Verification items for the finished model (mm, model axes). Face numbers are marked on the shaded views. A direction names the side the tool comes from. Round coordinates to 2 decimals unless told otherwise and drop trailing zeros. Order: outer loops, then holes, each group sorted by start corner. A loop starts at its lowest first (then second) coordinate and runs counter-clockwise, first axis right, second up. Notation, with made-up numbers: (80, -39) -> (94, -39) arc R16 ccw to (94, -31) -> close; hole circle Ø5 at (-37, -11.75). An arc over 180 degrees is marked (long way). Return JSON: item names as keys, results as strings. Group by question number.
Item 1: Sectioned sample at C-C on x = 19.5. Record the cut outline in (y, z), plus the area to 3 significant figures.
Item 2: Depth check by flat-ended pin: pin 1 Ø1.4 at (x, y) = (17.46, 17.65) entering from -Z (3 decimals); pin 2 Ø2 at (x, z) = (8, 2.5) entering from -Y; pin 3 Ø3 at (x, y) = (6, 12.5) entering from -Z; pin 4 Ø1 at (x, z) = (19.5, 4) entering from -Y. Enter the tip coordinate at first touch or a pass-through.
Item 3: Sectioned sample at B-B on y = 11.75. Record the cut outline in (x, z).
Item 4: Scan lines: probe 1 along Y at (x, z) = (15.5, 1.85); probe 2 along Y at (x, z) = (18, 1.4); probe 3 along X at (y, z) = (11.75, 3.35). Record each from-to range of solid material in increasing order. Write a range as from..to.
Item 5: Access from +Z, -Z, +X, -X, +Y, -Y to the whole of each face (thin tool, end or side, straight path). Record for the marked faces 1, 2 and 3.
Item 6: Sectioned sample at D-D on y = 18.75. Record the cut outline in (x, z), plus the area to 3 significant figures.
Item 7: Sectioned sample at A-A on z = 1.45. Record the cut outline in (x, y).
Item 8: Draft check along Y on the marked faces 4, 5, 6 and 7. Enter one of: pulls with the +Y half, pulls with the -Y half, needs draft (parallel to the pull), parting line crosses it, or undercut.
```python
from build123d import *

# Parameters (mm, degrees)
BOSS_EXTRUDE1_DEPTH = 5
SKETCH3_R           = 2.75
JOINT_HOLE_DEPTH    = 32.253054869
CUT_EXTRUDE2_START  = 0.5
CUT_EXTRUDE2_DEPTH  = 5.5
SKETCH7_R           = 0.8
SCREW_HOLES_DEPTH   = 32.253054869
BOSS_EXTRUDE2_START = 5
SKETCH10_W          = 3.875984902
SKETCH10_H          = 3
BOSS_EXTRUDE2_DEPTH = 0.5


with BuildPart() as part:
    # Sketch1 → Boss-Extrude1 (new body)
    with BuildSketch(Plane.XY):
        with BuildLine():
            Line((22.456085085, 19.15366827), (11.355064571, 19.15366827))
            ThreePointArc((11.355064571, 19.15366827), (-0.543914915, 14.15366827), (11.355064571, 9.15366827))
            Line((11.355064571, 9.15366827), (22.456085085, 9.15366827))
            Line((22.456085085, 9.15366827), (22.456085085, 19.15366827))
        make_face()
    extrude(amount=BOSS_EXTRUDE1_DEPTH)

    # Sketch3 → Joint Hole (cut, through all)
    with BuildSketch(Plane.XY):
        with Locations((6.456085085, 14.15366827)):
            Circle(SKETCH3_R)
    extrude(amount=JOINT_HOLE_DEPTH, mode=Mode.SUBTRACT)

    # Sketch8 → Cut-Extrude2 (cut)
    with BuildSketch(Plane.XY.offset(CUT_EXTRUDE2_START)):
        with BuildLine():
            Line((15.231049473, 12.15366827), (22.456085085, 12.15366827))
            Line((22.456085085, 12.15366827), (22.456085085, 16.15366827))
            Line((22.456085085, 16.15366827), (15.231049473, 16.15366827))
            ThreePointArc((15.231049473, 16.15366827), (14.722457344, 17.712753782), (13.939399859, 19.15366827))
            Line((13.939399859, 19.15366827), (11.355064571, 19.15366827))
            ThreePointArc((11.355064571, 19.15366827), (13.456085085, 14.15366827), (11.355064571, 9.15366827))
            Line((11.355064571, 9.15366827), (13.939399859, 9.15366827))
            ThreePointArc((13.939399859, 9.15366827), (14.722457344, 10.594582758), (15.231049473, 12.15366827))
        make_face()
    extrude(amount=CUT_EXTRUDE2_DEPTH, mode=Mode.SUBTRACT)

    # Sketch7 → Screw Holes (cut, through all)
    with BuildSketch(Plane.XY):
        with Locations((17.456085085, 17.65366827)):
            Circle(SKETCH7_R)
        with Locations((17.456085085, 10.65366827)):
            Circle(SKETCH7_R)
    extrude(amount=SCREW_HOLES_DEPTH, mode=Mode.SUBTRACT)

    # Sketch10 → Boss-Extrude2 (add)
    with BuildSketch(Plane.XY.offset(BOSS_EXTRUDE2_START)):
        with Locations((13.293057022, 17.65366827)):
            Rectangle(SKETCH10_W, SKETCH10_H)
        with Locations((13.293057022, 10.65366827)):
            Rectangle(SKETCH10_W, SKETCH10_H)
    extrude(amount=-BOSS_EXTRUDE2_DEPTH)


solid = part.part
```
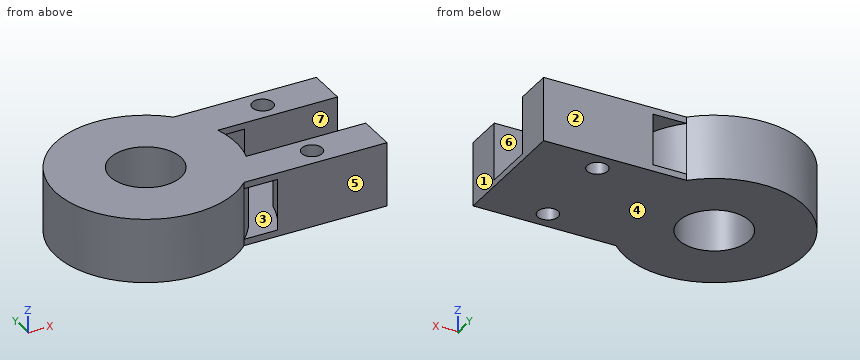
Recorded:
{
 "1": {"outline": "(9.15, 0) -> (19.15, 0) -> (19.15, 5) -> (16.15, 5) -> (16.15, 0.5) -> (12.15, 0.5) -> (12.15, 5) -> (9.15, 5) -> close", "area": "32.0 mm²"},
 "2": {"pin 1": "through", "pin 2": "y = 7.17", "pin 3": "z = 0", "pin 4": "y = 9.15"},
 "3": {"outline": "(-0.12, 0) -> (5.12, 0) -> (5.12, 5) -> (-0.12, 5) -> close; (7.79, 0) -> (22.46, 0) -> (22.46, 5) -> (7.79, 5) -> close; hole (13.03, 0.5) -> (15.13, 0.5) -> (15.13, 4.5) -> (13.03, 4.5) -> close"},
 "4": {"probe 1": "9.15..12.15, 16.15..19.15", "probe 2": "9.15..10.07, 11.24..12.15, 16.15..17.07, 18.24..19.15", "probe 3": "-0.12..5.12, 7.79..13.03, 15.13..22.46"},
 "5": {"face 1": "+Z, -Z, +X, +Y, -Y", "face 2": "+Z, -Z, +X, +Y", "face 3": "none"},
 "6": {"outline": "(1.18, 0) -> (22.46, 0) -> (22.46, 5) -> (1.18, 5) -> close; hole (11.74, 0.5) -> (14.19, 0.5) -> (14.19, 4.5) -> (11.74, 4.5) -> close", "area": "96.6 mm²"},
 "7": {"outline": "circle Ø14 at (6.46, 14.15); (13.94, 9.15) -> (22.46, 9.15) -> (22.46, 12.15) -> (15.23, 12.15) arc R9 cw to start; (13.94, 19.15) arc R9 cw to (15.23, 16.15) -> (22.46, 16.15) -> (22.46, 19.15) -> close; hole circle Ø5.5 at (6.46, 14.15); hole circle Ø1.6 at (17.46, 10.65); hole circle Ø1.6 at (17.46, 17.65)"},
 "8": {"face 4": "needs draft", "face 5": "pulls with the -Y half", "face 6": "undercut", "face 7": "undercut"}
}
